```python
from build123d import *

# Parameters (mm, degrees)
SKETCH1_W               = 200
SKETCH1_H               = 250
BOSS_EXTRUDE1_DEPTH     = 6
F_3_0MM_DOWEL_HOLE1_D   = 3.5
SKETCH6_R               = 1.75
CUT_EXTRUDE3_DEPTH      = 2.2
SKETCH2_W               = 200
SKETCH2_H               = 253.519525226
CUT_EXTRUDE2_DEPTH      = 1
CUT_EXTRUDE2_DEPTH_BACK = 7
BOSS_EXTRUDE3_DEPTH     = 6
SKETCH13_R              = 1.5
CUT_EXTRUDE4_DEPTH      = 1.0000001
CUT_EXTRUDE4_DEPTH_BACK = 7.0000001


with BuildPart() as part:
    # Sketch1 → Boss-Extrude1 (new body)
    with BuildSketch(Plane(origin=(0, 0, 0), x_dir=(1, 0, 0), z_dir=(0, 1, 0))):
        with Locations((100, 125)):
            Rectangle(SKETCH1_W, SKETCH1_H)
    extrude(amount=BOSS_EXTRUDE1_DEPTH)

    # Ø3.0mm Dowel Hole1 (through all)
    with Locations(Plane(origin=(0, 0, 0), x_dir=(-1, 0, 0), z_dir=(0, -1, 0))):
        with Locations((-83.29683767, 150.137900155), (-94.867014644, 163.926700131), (-121.29683767, 163.926700131), (-132.867014644, 150.137900155), (-128.081926157, 178.292602477), (-142.402815019, 169.888052337), (-88.081926157, 178.292602477), (-73.761037294, 169.888052337), (-133.867014644, 43.137900155), (-122.081926157, 40.922048355), (-122.29683767, 29.349100179), (-94.081926157, 40.922048355), (-93.867014644, 29.349100179), (-82.29683767, 43.137900155), (-72.761037294, 23.387747973), (-143.402815019, 23.387747973)):
            Hole(F_3_0MM_DOWEL_HOLE1_D / 2)

    # Sketch6 → Cut-Extrude3 (cut)
    with BuildSketch(Plane.XZ):
        Polygon((125.09683767, -27.732519425), (122.29683767, -26.115938672), (119.49683767, -27.732519425), (119.49683767, -30.965680933), (122.29683767, -32.582261686), (125.09683767, -30.965680933), align=None)
        Polygon((133.867014644, -39.904738648), (131.067014644, -41.521319401), (131.067014644, -44.754480909), (133.867014644, -46.371061663), (136.667014644, -44.754480909), (136.667014644, -41.521319401), align=None)
        Polygon((82.29683767, -39.904738648), (79.49683767, -41.521319401), (79.49683767, -44.754480909), (82.29683767, -46.371061663), (85.09683767, -44.754480909), (85.09683767, -41.521319401), align=None)
        Polygon((93.867014644, -26.115938672), (91.067014644, -27.732519425), (91.067014644, -30.965680933), (93.867014644, -32.582261686), (96.667014644, -30.965680933), (96.667014644, -27.732519425), align=None)
        Polygon((94.867014644, -160.693538624), (92.067014644, -162.310119378), (92.067014644, -165.543280885), (94.867014644, -167.159861639), (97.667014644, -165.543280885), (97.667014644, -162.310119378), align=None)
        with Locations((94.867014644, -163.926700131)):
            Circle(SKETCH6_R, mode=Mode.SUBTRACT)
        Polygon((83.29683767, -146.904738648), (80.49683767, -148.521319401), (80.49683767, -151.754480909), (83.29683767, -153.371061663), (86.09683767, -151.754480909), (86.09683767, -148.521319401), align=None)
        with Locations((83.29683767, -150.137900155)):
            Circle(SKETCH6_R, mode=Mode.SUBTRACT)
        Polygon((121.29683767, -160.693538624), (118.49683767, -162.310119378), (118.49683767, -165.543280885), (121.29683767, -167.159861639), (124.09683767, -165.543280885), (124.09683767, -162.310119378), align=None)
        with Locations((121.29683767, -163.926700131)):
            Circle(SKETCH6_R, mode=Mode.SUBTRACT)
        Polygon((132.867014644, -153.371061663), (135.667014644, -151.754480909), (135.667014644, -148.521319401), (132.867014644, -146.904738648), (130.067014644, -148.521319401), (130.067014644, -151.754480909), align=None)
        with Locations((132.867014644, -150.137900155)):
            Circle(SKETCH6_R, mode=Mode.SUBTRACT)
    extrude(amount=-CUT_EXTRUDE3_DEPTH, mode=Mode.SUBTRACT)

    # Sketch2 → Cut-Extrude2 (cut, two sides)
    with BuildSketch(Plane.XZ) as cut_extrude2_sk:
        with Locations((100, -126.759762613)):
            Rectangle(SKETCH2_W, SKETCH2_H)
        with BuildLine():
            Line((143.206271193, -38.474324409), (139.348594785, -82.567767518))
            ThreePointArc((139.348594785, -82.567767518), (143.379983208, -88.766434624), (138.333453387, -94.170886794))
            Line((138.333453387, -94.170886794), (138.081926157, -97.045856194))
            Line((138.081926157, -97.045856194), (140.863131926, -149.832051752))
            ThreePointArc((140.863131926, -149.832051752), (142.359866063, -154.590769387), (145.969242496, -158.034315287))
            Line((145.969242496, -158.034315287), (156.230851695, -163.771558937))
            Line((156.230851695, -163.771558937), (144.440739957, -184.859301843))
            add(Edge.make_bspline(
                [(144.440739957, -184.859301843), (137.686448173, -178.410982542), (137.402815019, -190.036315102)],
                knots=[0, 0, 0, 1, 1, 1], degree=2))
            Line((137.402815019, -190.036315102), (78.761037294, -190.036315102))
            add(Edge.make_bspline(
                [(71.723112356, -184.859301843), (78.47740414, -178.410982542), (78.761037294, -190.036315102)],
                knots=[0, 0, 0, 1, 1, 1], degree=2))
            Line((71.723112356, -184.859301843), (59.933000618, -163.771558937))
            Line((59.933000618, -163.771558937), (70.194609818, -158.034315287))
            ThreePointArc((70.194609818, -158.034315287), (73.803986251, -154.590769387), (75.300720388, -149.832051752))
            Line((75.300720388, -149.832051752), (78.081926157, -97.045856194))
            Line((78.081926157, -97.045856194), (77.830398926, -94.170886794))
            ThreePointArc((77.830398926, -94.170886794), (72.783869106, -88.766434624), (76.815257528, -82.567767518))
            Line((76.815257528, -82.567767518), (72.95758112, -38.474324409))
            add(Edge.make_bspline(
                [(71.87426297, -36.548342356), (73.029938343, -36.460716162), (72.980934293, -37.754807476), (72.95758112, -38.474324409)],
                knots=[0, 0, 0, 0, 1, 1, 1, 1], degree=3))
            Line((71.87426297, -36.548342356), (65.214123879, -34.172936949))
            Line((65.214123879, -34.172936949), (56.844705507, -27.15016108))
            Line((56.844705507, -27.15016108), (73.702448882, -7.059884849))
            Line((73.702448882, -7.059884849), (82.071867254, -14.082660719))
            add(Edge.make_bspline(
                [(82.071867254, -14.082660719), (83.53149801, -15.797125086), (85.909052418, -16.455495951), (88.081926157, -16.243500167)],
                knots=[0, 0, 0, 0, 1, 1, 1, 1], degree=3))
            Line((88.081926157, -16.243500167), (128.081926157, -16.243500167))
            add(Edge.make_bspline(
                [(134.09198506, -14.082660719), (132.632354304, -15.797125086), (130.254799895, -16.455495951), (128.081926157, -16.243500167)],
                knots=[0, 0, 0, 0, 1, 1, 1, 1], degree=3))
            Line((134.09198506, -14.082660719), (142.461403432, -7.059884849))
            Line((142.461403432, -7.059884849), (159.319146807, -27.15016108))
            Line((159.319146807, -27.15016108), (150.949728435, -34.172936949))
            Line((150.949728435, -34.172936949), (144.289589344, -36.548342356))
            add(Edge.make_bspline(
                [(144.289589344, -36.548342356), (143.133913971, -36.460716162), (143.182918021, -37.754807476), (143.206271193, -38.474324409)],
                knots=[0, 0, 0, 0, 1, 1, 1, 1], degree=3))
        make_face(mode=Mode.SUBTRACT)
    extrude(amount=CUT_EXTRUDE2_DEPTH, mode=Mode.SUBTRACT)
    extrude(cut_extrude2_sk.sketch, amount=-CUT_EXTRUDE2_DEPTH_BACK, mode=Mode.SUBTRACT)

    # Sketch12 → Boss-Extrude3 (add)
    with BuildSketch(Plane.XZ):
        with BuildLine():
            Line((145.333785649, -131.181364351), (145.333785649, -77.629044584))
            add(Edge.make_bspline(
                [(147.619658889, -35.360639653), (142.777206683, -37.926752291), (144.388952605, -55.69848949), (143.790680066, -63.416837485), (144.241351516, -74.545098791), (145.333785649, -77.629044584)],
                knots=[0, 0, 0, 0, 0.389986275, 0.710398556, 0.928445879, 0.928445879, 0.928445879, 0.928445879], degree=3))
            Line((147.619658889, -35.360639653), (144.289589344, -36.548342356))
            add(Edge.make_bspline(
                [(143.206271193, -38.474324409), (143.182918021, -37.754807476), (143.133913971, -36.460716162), (144.289589344, -36.548342356)],
                knots=[0, 0, 0, 0, 1, 1, 1, 1], degree=3))
            Line((143.206271193, -38.474324409), (139.348594785, -82.567767518))
            ThreePointArc((139.348594785, -82.567767518), (143.379983208, -88.766434624), (138.333453387, -94.170886794))
            Line((138.333453387, -94.170886794), (138.081926157, -97.045856194))
            Line((138.081926157, -97.045856194), (140.863131926, -149.832051752))
            ThreePointArc((140.863131926, -149.832051752), (142.359866063, -154.590769387), (145.969242496, -158.034315287))
            Line((145.969242496, -158.034315287), (151.100047096, -160.902937112))
            add(Edge.make_bspline(
                [(151.100047096, -160.902937112), (144.231308287, -154.695867795), (145.4211977, -148.853665316), (144.801008685, -133.708262299), (145.333785649, -131.181364351)],
                knots=[0, 0, 0, 0, 0.606254863, 0.822010641, 0.822010641, 0.822010641, 0.822010641], degree=3))
        make_face()
        with BuildLine():
            Line((70.830066664, -131.181364351), (70.830066664, -77.629044584))
            add(Edge.make_bspline(
                [(68.544193424, -35.360639653), (73.38664563, -37.926752291), (71.774899708, -55.69848949), (72.373172248, -63.416837485), (71.922500798, -74.545098791), (70.830066664, -77.629044584)],
                knots=[0, 0, 0, 0, 0.389986275, 0.710398556, 0.928445879, 0.928445879, 0.928445879, 0.928445879], degree=3))
            Line((68.544193424, -35.360639653), (71.87426297, -36.548342356))
            add(Edge.make_bspline(
                [(72.95758112, -38.474324409), (72.980934293, -37.754807476), (73.029938343, -36.460716162), (71.87426297, -36.548342356)],
                knots=[0, 0, 0, 0, 1, 1, 1, 1], degree=3))
            Line((72.95758112, -38.474324409), (76.815257528, -82.567767518))
            ThreePointArc((76.815257528, -82.567767518), (72.783869106, -88.766434624), (77.830398926, -94.170886794))
            Line((77.830398926, -94.170886794), (78.081926157, -97.045856194))
            Line((78.081926157, -97.045856194), (75.300720388, -149.832051752))
            ThreePointArc((75.300720388, -149.832051752), (73.803986251, -154.590769387), (70.194609818, -158.034315287))
            Line((70.194609818, -158.034315287), (65.063805218, -160.902937112))
            add(Edge.make_bspline(
                [(65.063805218, -160.902937112), (71.932544027, -154.695867795), (70.742654614, -148.853665316), (71.362843629, -133.708262299), (70.830066664, -131.181364351)],
                knots=[0, 0, 0, 0, 0.606254863, 0.822010641, 0.822010641, 0.822010641, 0.822010641], degree=3))
        make_face()
    extrude(amount=-BOSS_EXTRUDE3_DEPTH)

    # Sketch13 → Cut-Extrude4 (cut, two sides)
    with BuildSketch(Plane.XZ) as cut_extrude4_sk:
        with Locations((139.6953643, -52.871061663)):
            Circle(SKETCH13_R)
        with Locations((76.6953643, -52.871061663)):
            Circle(SKETCH13_R)
        with Locations((76.6953643, -139.871061663)):
            Circle(SKETCH13_R)
        with Locations((139.6953643, -139.871061663)):
            Circle(SKETCH13_R)
    extrude(amount=CUT_EXTRUDE4_DEPTH, mode=Mode.SUBTRACT)
    extrude(cut_extrude4_sk.sketch, amount=-CUT_EXTRUDE4_DEPTH_BACK, mode=Mode.SUBTRACT)


solid = part.part
```
The model under review builds one solid part; all positions refer to its coordinate system, in mm. A direction names the side the tool comes from. Coordinates: 2 decimals unless noted, no trailing zeros. Write each loop counter-clockwise with the first axis right and the second up, starting at its lowest first coordinate (ties: lowest second). Pieces come first, ordered by that corner, then holes. Notation, with made-up numbers: (88.5, 72) - (109.5, 72) arc R21 cw to (109.5, 111) - close; hole circle Ø9 at (26, -35). An arc over 180 degrees is marked (long way). Answer in a Markdown table with one row per item. Add a question column.
Q1. Consider section B-B on y = 1. Give the number of separate pieces and of enclosed holes in the cut face, then the cut area to 3 significant figures.
Q2. Draft analysis for pull direction X (two halves, no side actions). For faces 1 (the face through (153.6, 3, -162.3)), 2 (the face through (65.91, 2.96, -174.46)), 3 (the face through (133, 2.2, -45)), state which applies: +X half, -X half, draft (parallel to the pull), parting line (faces both ways), or undercut.
Q3. Consider section A-A on z = -79.5. Give the boundary of the cut face in (x, y).
Q4. For faces 4 (the face through (145.334, 3, -105)), 5 (the face through (62.46, 2.96, -162.36)), 6 (the face through (108, 3, -16.244)), 7 (the face through (145.072, 3.042, -23.913)), 8 (the face through (95, 2.2, -31)), list the 3-axis set-ups (+Z, -Z, +X, -X, +Y, -Y) from which the entire face can be reached by the end or side of a thin tool; tool diameter is ignored.
Q5. To check wall thickness, follow line 1 along Z through (x, y) = (135.5, 1.75); line 2 along X through (y, z) = (5.5, -52.5); line 3 along Z through (x, y) = (112.5, 4.5). State the ranges of each line that lie inside material, in increasing order. Write a range as from..to.
Q6. Clearance check with flat-ended pins moving along their axes: pin 1 (1.7 mm diameter, centred on x = 133.5, z = -43, fed in from -Y); pin 2 (2.5 mm diameter, centred on y = 1, z = -30, fed in from +X); pin 3 (4 mm diameter, centred on x = 82.3, z = -43.14, fed in from -Y); pin 4 (0.7 mm diameter, centred on y = 1, z = -30, fed in from +X). State where each tip first meets the part, or that it passes through.
Q7. Consider section C-C on x = 115.5. Give the boundary of the cut face in (y, z), then the cut area to 3 significant figures.
Answers below:
| question | item | result |
|---|---|---|
| 1 | separate pieces | 1 |
| 1 | enclosed holes | 20 |
| 1 | area | 13,200 mm² |
| 2 | face 1 | +X half |
| 2 | face 2 | -X half |
| 2 | face 3 | undercut |
| 3 | outline | (70.83, 0) - (145.33, 0) - (145.33, 6) - (70.83, 6) - close |
| 4 | face 4 | +X, +Y, -Y |
| 4 | face 5 | -X, +Y, -Y |
| 4 | face 6 | +Z, +Y, -Y |
| 4 | face 7 | +Y, -Y |
| 4 | face 8 | -Y |
| 5 | line 1 | -190.04..-151.85, -148.42..-45.43, -40.85..-12.9 |
| 5 | line 2 | 72.3..75.24, 78.15..138.24, 141.15..143.86 |
| 5 | line 3 | -190.04..-16.24 |
| 6 | pin 1 | through |
| 6 | pin 2 | x = 157.41 |
| 6 | pin 3 | y = 2.2 |
| 6 | pin 4 | x = 156.34 |
| 7 | outline | (0, -190.04) - (6, -190.04) - (6, -16.24) - (0, -16.24) - close |
| 7 | area | 1,040 mm² |
